```python
from build123d import *

# Parameters (mm, degrees)
SKETCH1_R               = 2.5273
BOSS_EXTRUDE2_DEPTH     = 9.398
BOSS_EXTRUDE3_DEPTH     = 1.524
BOSS_EXTRUDE4_DEPTH     = 1.5875
SKETCH4_W               = 12.7
SKETCH4_H               = 9.525
CUT_EXTRUDE1_DEPTH      = 56.4355
CUT_EXTRUDE1_DEPTH_BACK = 56.4355


with BuildPart() as part:
    # Sketch1 → Boss-Extrude2 (new body, symmetric)
    with BuildSketch(Plane(origin=(0, 0, 0), x_dir=(0, 0, -1), z_dir=(1, 0, 0))):
        Polygon((-6.35, -45.9105), (6.35, -45.9105), (6.35, 45.9105), (-6.35, 45.9105), (-31.75, 45.9105), (-31.75, 42.8625), (-6.35, 42.8625), (-6.35, 39.8145), (-31.75, 39.8145), (-31.75, 36.7665), (-6.35, 36.7665), (-6.35, -36.7665), (-31.75, -36.7665), (-31.75, -39.8145), (-6.35, -39.8145), (-6.35, -42.8625), (-31.75, -42.8625), (-31.75, -45.9105), align=None)
        with Locations((1.5875, 36.3855)):
            Circle(SKETCH1_R, mode=Mode.SUBTRACT)
        with Locations((1.5875, -36.3855)):
            Circle(SKETCH1_R, mode=Mode.SUBTRACT)
    extrude(amount=BOSS_EXTRUDE2_DEPTH, both=True)

    # Sketch2 → Boss-Extrude3 (add, symmetric)
    with BuildSketch(Plane(origin=(0, 0, 0), x_dir=(0, 0, -1), z_dir=(1, 0, 0))):
        Polygon((-8.89, 55.4355), (-3.81, 50.3555), (-3.81, 45.9105), (-31.75, 45.9105), (-31.75, 55.4355), align=None)
        Polygon((-31.75, -45.9105), (-31.75, -55.4355), (-8.89, -55.4355), (-3.81, -50.3555), (-3.81, -45.9105), align=None)
    extrude(amount=BOSS_EXTRUDE3_DEPTH, both=True)

    # Sketch3 → Boss-Extrude4 (add, symmetric)
    with BuildSketch(Plane(origin=(0, 0, 0), x_dir=(0, 0, -1), z_dir=(1, 0, 0))):
        Polygon((-19.820384182, 36.7665), (-6.35, 23.296115818), (-6.35, 36.7665), align=None)
        Polygon((-19.820384182, -36.7665), (-6.35, -36.7665), (-6.35, -23.296115818), align=None)
    extrude(amount=BOSS_EXTRUDE4_DEPTH, both=True)

    # Sketch4 → Cut-Extrude1 (cut, two sides)
    with BuildSketch(Plane(origin=(0, 0, 0), x_dir=(1, 0, 0), z_dir=(0, 1, 0))) as cut_extrude1_sk:
        with Locations((0, 1.5875)):
            Rectangle(SKETCH4_W, SKETCH4_H)
    extrude(amount=CUT_EXTRUDE1_DEPTH, mode=Mode.SUBTRACT)
    extrude(cut_extrude1_sk.sketch, amount=-CUT_EXTRUDE1_DEPTH_BACK, mode=Mode.SUBTRACT)


solid = part.part
```
Can you work these out from the model? Positions are in its coordinate system, mm. A direction names the side the tool comes from. Coordinates: 2 decimals unless noted, no trailing zeros. Order: outer loops, then holes, each group sorted by start corner. A loop starts at its lowest first (then second) coordinate and runs counter-clockwise, first axis right, second up.
1. I'm going to push flat-ended pins straight in: pin 1 (4 mm diameter, centred on y = 33, z = 14, fed in from +X); pin 2 (1.5 mm diameter, centred on x = -4.5, z = 5.5, fed in from -Y); pin 3 (1.5 mm diameter, centred on x = -2, y = -41, fed in from +Z). Where does each tip first touch, or does it pass through?
2. For faces 4 (the face through (-1.588, -33, 10)), 5 (the face through (0, 48, 3.81)), 6 (the face through (0.022, -29.937, 12.991)), 7 (the face through (-1.524, 51, 18)), which set-ups out of +Z, -Z, +X, -X, +Y, -Y let a thin tool reach every point of the face, with its end or its side?
3. If we section it at A-A (z = 28): Please give me the cut outline in (x, y).
4. Thinking about a two-plate mould opening in Y: for faces 1 (the face through (1.588, 33, 10)), 2 (the face through (0, 55.436, 20)), 3 (the face through (1.524, 51, 18)), which applies, +Y half, -Y half, draft (parallel to the pull), parting line (faces both ways), or undercut?
5. If we section it at D-D (y = 1.5): Please give me the cut outline in (x, z) (3 decimals).
6. If we section it at C-C (z = -1.5): Please give me the cut outline in (x, y), then the cut area to 3 significant figures.
7. I need wall thicknesses on line 1 (Y direction, x = 8.5, z = 11); line 2 (X direction, y = 6.5, z = 2); line 3 (Y direction, x = 8, z = -0.5). Which ranges of each line are inside material? Lowest first, please.
Entries:
1. pin 1: stops at x = 1.59
1. pin 2: stops at y = -45.91
1. pin 3: stops at z = 6.35
2. face 4: +Z, -X
2. face 5: -Z, +X, -X, +Y
2. face 6: +Z, +X, -X
2. face 7: +Z, -Z, -X, +Y
3. outline: (-9.4, -45.91) - (-1.52, -45.91) - (-1.52, -55.44) - (1.52, -55.44) - (1.52, -45.91) - (9.4, -45.91) - (9.4, -42.86) - (-9.4, -42.86) - close; (-9.4, -39.81) - (9.4, -39.81) - (9.4, -36.77) - (-9.4, -36.77) - close; (-9.4, 36.77) - (9.4, 36.77) - (9.4, 39.81) - (-9.4, 39.81) - close; (-9.4, 42.86) - (9.4, 42.86) - (9.4, 45.91) - (1.52, 45.91) - (1.52, 55.44) - (-1.52, 55.44) - (-1.52, 45.91) - (-9.4, 45.91) - close
4. face 1: undercut
4. face 2: +Y half
4. face 3: draft
5. outline: (-9.398, -6.35) - (-6.35, -6.35) - (-6.35, 3.175) - (6.35, 3.175) - (6.35, -6.35) - (9.398, -6.35) - (9.398, 6.35) - (-9.398, 6.35) - close
6. outline: (-9.4, -45.91) - (-6.35, -45.91) - (-6.35, -38.91) - (-9.4, -38.91) - close; (-9.4, -33.86) - (-6.35, -33.86) - (-6.35, 33.86) - (-9.4, 33.86) - close; (-9.4, 38.91) - (-6.35, 38.91) - (-6.35, 45.91) - (-9.4, 45.91) - close; (6.35, -45.91) - (9.4, -45.91) - (9.4, -38.91) - (6.35, -38.91) - close; (6.35, -33.86) - (9.4, -33.86) - (9.4, 33.86) - (6.35, 33.86) - close; (6.35, 38.91) - (9.4, 38.91) - (9.4, 45.91) - (6.35, 45.91) - close
6. area: 498 mm2
7. line 1: y = -45.91 to -42.86, -39.81 to -36.77, 36.77 to 39.81, 42.86 to 45.91
7. line 2: x = -9.4 to -6.35, 6.35 to 9.4
7. line 3: y = -45.91 to -38.67, -34.1 to 34.1, 38.67 to 45.91
